from build123d import *

# Parameters (mm, degrees)
BOSS_EXTRUDE1_DEPTH      = 2.5
BOSS_EXTRUDE1_DEPTH_BACK = 2.5
SKETCH3_R                = 60
BOSS_EXTRUDE2_DEPTH      = 6
BOSS_EXTRUDE2_DEPTH_BACK = 11
SKETCH4_R                = 28.5
BOSS_EXTRUDE5_DEPTH      = 45
FILLET4_R                = 25
SKETCH5_R                = 24
CUT_EXTRUDE2_DEPTH       = 37


with BuildPart() as part:
    # Sketch1 → Boss-Extrude1 (new body, two sides)
    with BuildSketch(Plane(origin=(0, 0, 0), x_dir=(1, 0, 0), z_dir=(0, 1, 0))) as boss_extrude1_sk:
        with BuildLine():
            ThreePointArc((-50.816530808, 31.901100241), (-56.123031071, 21.218043817), (-59.211320918, 9.696364016))
            add(Edge.make_bspline(
                [(-2.218897813, -59.958956733), (-433.653695627, -354.818191007), (-59.211320918, 9.696364016)],
                knots=[0, 0, 0, 1, 1, 1], degree=2))
            ThreePointArc((-2.218897813, -59.958956733), (9.686150572, -59.212992553), (21.208362897, -56.126690115))
            add(Edge.make_bspline(
                [(53.035428622, 28.057856492), (524.108414951, -198.146021355), (21.208362897, -56.126690115)],
                knots=[0, 0, 0, 1, 1, 1], degree=2))
            ThreePointArc((53.035428622, 28.057856492), (46.436880499, 37.994948737), (38.002958021, 46.430326099))
            add(Edge.make_bspline(
                [(-50.816530808, 31.901100241), (-90.454719323, 552.964212362), (38.002958021, 46.430326099)],
                knots=[0, 0, 0, 1, 1, 1], degree=2))
        make_face()
    extrude(amount=BOSS_EXTRUDE1_DEPTH)
    extrude(boss_extrude1_sk.sketch, amount=-BOSS_EXTRUDE1_DEPTH_BACK)

    # Sketch3 → Boss-Extrude2 (add, two sides)
    with BuildSketch(Plane(origin=(0, 2.5, 0), x_dir=(1, 0, 0), z_dir=(0, 1, 0))) as boss_extrude2_sk:
        Circle(SKETCH3_R)
    extrude(amount=BOSS_EXTRUDE2_DEPTH)
    extrude(boss_extrude2_sk.sketch, amount=-BOSS_EXTRUDE2_DEPTH_BACK)

    # Sketch4 → Boss-Extrude5 (add)
    with BuildSketch(Plane(origin=(0, 8.5, 0), x_dir=(1, 0, 0), z_dir=(0, 1, 0))):
        Circle(SKETCH4_R)
    extrude(amount=BOSS_EXTRUDE5_DEPTH)

    # Fillet4
    fillet4_edges = [part.edges().sort_by_distance(p)[0] for p in [
        (-28.5, 53.5, 0),
    ]]
    fillet(fillet4_edges, radius=FILLET4_R)

    # Sketch5 → Cut-Extrude2 (cut)
    with BuildSketch(Plane.XZ.offset(8.5)):
        Circle(SKETCH5_R)
    extrude(amount=-CUT_EXTRUDE2_DEPTH, mode=Mode.SUBTRACT)


solid = part.part
Geometry: final body of the model. Coordinates: model frame, mm. A direction names the side the tool comes from. Give positions to 0.01 mm unless a question says otherwise; leave off trailing zeros. Loops run counter-clockwise (first coordinate to the right, second up) from the corner with the lowest first, then second, coordinate; pieces in that order, holes last. Notation, with made-up numbers: (37, 71) -> (81, 71) arc R28 cw to (81, 89) -> close; hole circle Ø10 at (29, -12). An arc over 180 degrees is marked (long way). Put each result on its own line as item: value.
1. Cut plane A-A (y = 18.5). Return the cut outline in (x, z).
Taken from the geometry:
outline: circle Ø57 at (0, 0); hole circle Ø48 at (0, 0)
2. Pull-direction query (Z, two-part tool) for faces 1 (the cylindrical face through (-23.977, 9.741, 1.055)), 2 (the flat face through (141, -2.5, 51)), 3 (the cylindrical face through (26.327, 18.36, 10.916)); classes: released by +Z, released by -Z, zero draft, split by the parting line, or undercut.
Taken from the geometry:
face 1: undercut
face 2: zero draft
face 3: split by the parting line
3. Ray query, line 1 along Z through (x, y) = (0, 9); line 2 along Y through (x, z) = (-41.5, -195); line 3 along X through (y, z) = (17, -19.5). Return the intervals inside material, ascending. Write a range as [from, to].
Taken from the geometry:
line 1: z = [-28.5, -24], [24, 28.5]
line 2: y = [-2.5, 2.5]
line 3: x = [-20.78, -13.99], [13.99, 20.78]
4. Pin query (flat end, axial travel): P1, Ø1.5, axis at y = 10, z = 3, coming from the -X side; P2, Ø14.5, axis at x = -5.5, z = -6, coming from the -Y side; P3, Ø3, axis at x = -156.5, y = 1, coming from the +Z side. Return the tip coordinate at first contact, or that it passes through.
Taken from the geometry:
P1: stops at x = -28.41
P2: stops at y = 28.5
P3: stops at z = 160.69
5. Set-up query: faces 4 (the flat face through (26, -8.5, -1)), 5 (the flat face through (-123, -2.5, 91)), 6 (the flat face through (0, 28.5, 0)), 7 (the flat face through (25.8, 8.5, 12.5)). Return all of +Z, -Z, +X, -X, +Y, -Y with unobstructed straight access to the full face (end or side cutting, diameter ignored); none if empty.
Taken from the geometry:
face 4: +Z, -Z, +X, -X, -Y
face 5: +Z, -X, -Y
face 6: -Y
face 7: +Y
